Could you check a few things on this model? Use its own coordinates, in mm. Face numbers are marked on the shaded views. A direction names the side the tool comes from. Coordinates: 2 decimals unless noted, no trailing zeros. Order: outer loops, then holes, each group sorted by start corner. A loop starts at its lowest first (then second) coordinate and runs counter-clockwise, first axis right, second up. Notation, with made-up numbers: (-32.5, 87.25) -> (22.5, 87.25) arc R15 ccw to (22.5, 97.25) -> close; hole circle Ø10 at (11.25, 43.5). An arc over 180 degrees is marked (long way). Use a Markdown table: item, result. Add a question column.
1) If we section it at C-C (x = 34.5): Give the number of separate pieces and of enclosed holes in the cut face, plus the area to 3 significant figures.
2) Which directions (+Z, -Z, +X, -X, +Y, -Y) give clear straight access to the entire face, cutting with the end or side of a thin tool? Please do the marked faces 3 and 4.
3) Thinking about a two-plate mould opening in X: for the marked faces 1 and 2, which applies, +X half, -X half, draft (parallel to the pull), parting line (faces both ways), or undercut?
4) If I drill on L1, parallel to Y at x = 34.5, z = -0.25; L2, parallel to Z at x = 23, y = -4.5; L3, parallel to X at y = 10.5, z = 4.75, over which ranges is the centre line in solid material (lowest first)? Write a range as [from, to].
5) Will these pins go through, and if not, where does the flat tip stop? pin 1 Ø4.5 at (x, y) = (-34.5, -34.5) entering from +Z; pin 2 Ø3 at (x, z) = (-30, 3) entering from +Y; pin 3 Ø5 at (y, z) = (9.5, 5.5) entering from -X.
6) If we section it at A-A (y = 0): Write out the boundary of the cut face in (x, z).
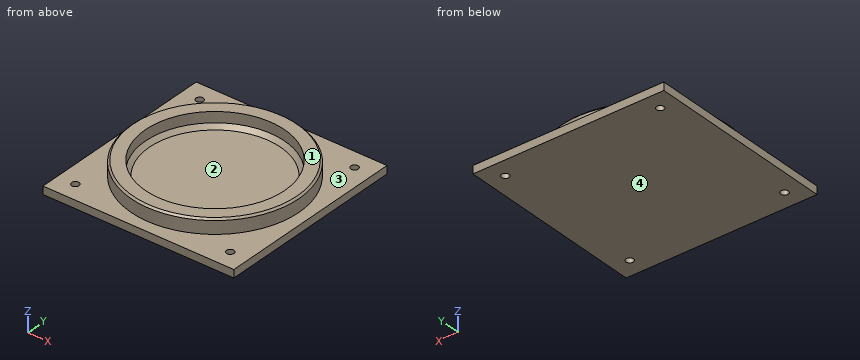
Solid Edge part; units mm, degrees
sketch "Sketch1" plane through (0, 0, 0) normal (0, 0, 1) x (1, 0, 0)
  circle A0 centre (34.5, 34.5) radius 1.65
  circle A1 centre (-34.5, 34.5) radius 1.65
  circle A2 centre (-34.5, -34.5) radius 1.65
  circle A3 centre (34.5, -34.5) radius 1.65
  line L0 (42.5, 42.5) -> (-42.5, 42.5)
  line L1 (-42.5, 42.5) -> (-42.5, -42.5)
  line L2 (-42.5, -42.5) -> (42.5, -42.5)
  line L3 (42.5, -42.5) -> (42.5, 42.5)
extrude "Protrusion1" add sketch "Sketch1" against normal blind 3.5
sketch "Sketch2" plane through (0, 0, 0) normal (0, 0, 1) x (1, 0, 0)
  circle A0 centre (0, 0) radius 31
  circle A1 centre (0, 0) radius 37.35
extrude "ExtrudedProtrusion_2" add sketch "Sketch2" along normal blind 6.5
chamfer "Chamfer_1" distance 0.8 angle 45 1 edges at (-37.35, 0, 6.5)
chamfer "Chamfer_2" distance 1.8 angle 45 1 edges at (-31, 0, 0)
Answer sheet:
| question | item | result |
|---|---|---|
| 1 | separate pieces | 3 |
| 1 | enclosed holes | 0 |
| 1 | area | 459 mm2 |
| 2 | face 3 | +Z |
| 2 | face 4 | -Z, +X, -X, +Y, -Y |
| 3 | face 1 | draft |
| 3 | face 2 | undercut |
| 4 | L1 | [-42.5, -36.15], [-32.85, 32.85], [36.15, 42.5] |
| 4 | L2 | [-3.5, 0] |
| 4 | L3 | [-35.84, -29.17], [29.17, 35.84] |
| 5 | pin 1 | z = 0 |
| 5 | pin 2 | y = 24.14 |
| 5 | pin 3 | x = -36.69 |
| 6 | outline | (-42.5, -3.5) -> (42.5, -3.5) -> (42.5, 0) -> (37.35, 0) -> (37.35, 5.7) -> (36.55, 6.5) -> (31, 6.5) -> (31, 1.8) -> (29.2, 0) -> (-29.2, 0) -> (-31, 1.8) -> (-31, 6.5) -> (-36.55, 6.5) -> (-37.35, 5.7) -> (-37.35, 0) -> (-42.5, 0) -> close |
